Here's the drawing with two shaded views (mm, measured from the low corner). I have some questions. A direction names the side the tool comes from. Give positions to 0.01 mm unless a question says otherwise; leave off trailing zeros. Write each loop counter-clockwise with the first axis right and the second up, starting at its lowest first coordinate (ties: lowest second). Pieces come first, ordered by that corner, then holes. Notation, with made-up numbers: (55.5, 26.25) -> (77.5, 26.25) arc R22 ccw to (77.5, 49.25) -> close; hole circle Ø1 at (44, 64.5). An arc over 180 degrees is marked (long way). One line per question, with ' | ' between items.
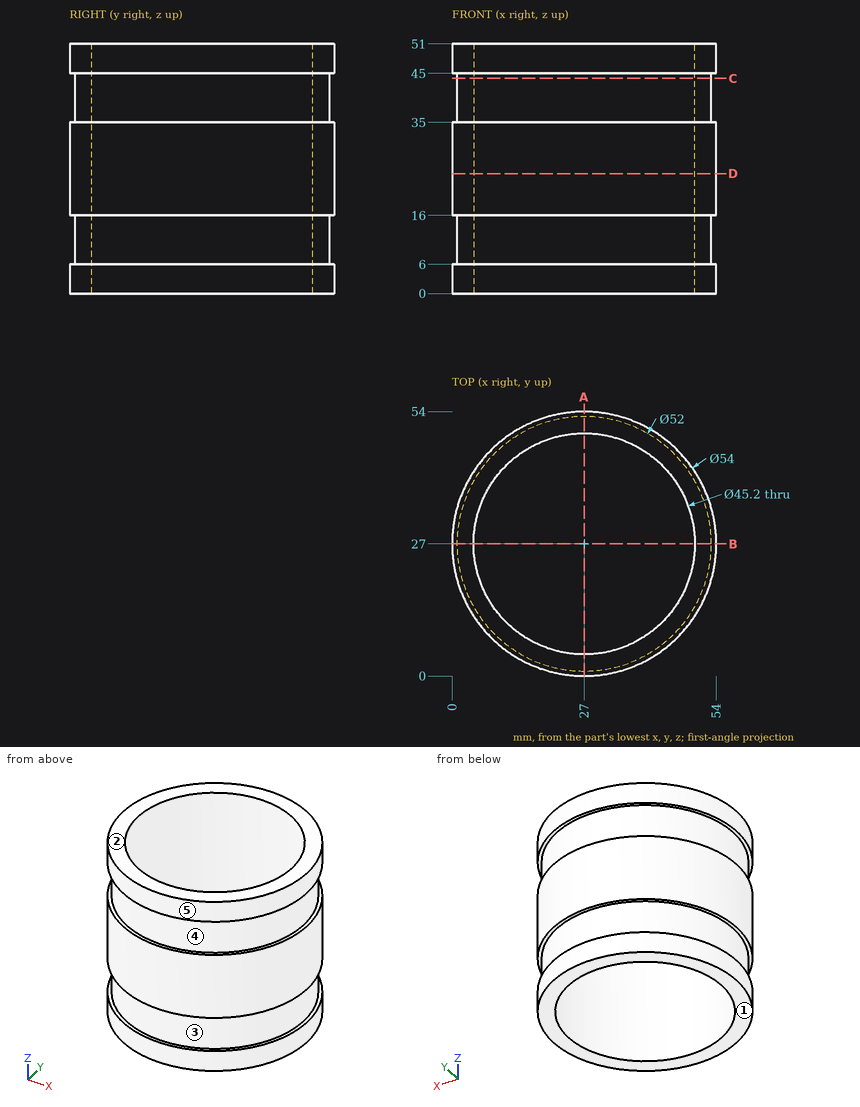
Q1. On a 3-axis mill with a long thin cutter (end or side, diameter ignored), from which of +Z, -Z, +X, -X, +Y, -Y can I reach the whole of each face in a straight line? I mean the marked faces 4 and 5. Say none if no direction works.
Answer below:
face 4: none | face 5: +Z, -Z
Q2. If I drill on line 1 along X through (y, z) = (26.5, 17); line 2 along Y through (x, z) = (27, 19); line 3 along X through (y, z) = (7, 37.5), over which ranges is the centre line in solid material (lowest first)?
Answer below:
line 1: x = 0 to 4.41, 49.59 to 54 | line 2: y = 0 to 4.4, 49.6 to 54 | line 3: x = 10.39 to 16.48, 37.52 to 43.61
Q3. Imagine slicing it at C-C on z = 44. Please give me the cut outline in (x, y).
Answer below:
outline: circle Ø52 at (27, 27); hole circle Ø45.2 at (27, 27)
Q4. Imagine slicing it at D-D on z = 24.5. Please give me the cut outline in (x, y).
Answer below:
outline: circle Ø54 at (27, 27); hole circle Ø45.2 at (27, 27)
Q5. Will these pins go through, and if not, where does the flat tip stop? pin 1 (1 mm diameter, centred on y = 35, z = 31, fed in from +X); pin 2 (1.5 mm diameter, centred on y = 10.5, z = 14.5, fed in from +X); pin 3 (3 mm diameter, centred on x = 6.5, z = 40.5, fed in from +Y).
Answer below:
pin 1: stops at x = 52.94 | pin 2: stops at x = 47.69 | pin 3: stops at y = 44.75
Q6. If we mould it in two halves opening along Z, with no side actions, what happens to the marked faces 1, 2 and 3? For each: +Z half, -Z half, draft (parallel to the pull), parting line (faces both ways), or undercut.
Answer below:
face 1: -Z half | face 2: +Z half | face 3: undercut
Q7. Imagine slicing it at A-A on x = 27. Please give me the cut outline in (y, z).
Answer below:
outline: (0, 0) -> (4.4, 0) -> (4.4, 51) -> (0, 51) -> (0, 45) -> (1, 45) -> (1, 35) -> (0, 35) -> (0, 16) -> (1, 16) -> (1, 6) -> (0, 6) -> close; (49.6, 0) -> (54, 0) -> (54, 6) -> (53, 6) -> (53, 16) -> (54, 16) -> (54, 35) -> (53, 35) -> (53, 45) -> (54, 45) -> (54, 51) -> (49.6, 51) -> close
